```python
from build123d import *

# Parameters (mm, degrees)
SKETCH_W     = 10
SKETCH_H     = 10
PAD_DEPTH    = 2
SKETCH001_W  = 10
SKETCH001_H  = 10
PAD001_DEPTH = 2
SKETCH002_R  = 2.45
PAD002_DEPTH = 3.8
FILLET_R     = 2


with BuildPart() as part:
    # Sketch → Pad (new body)
    with BuildSketch(Plane.XY):
        Rectangle(SKETCH_W, SKETCH_H)
    extrude(amount=PAD_DEPTH)

    # Sketch001 (on Face3 of Pad) → Pad001 (join)
    with BuildSketch(Plane.XZ.offset(5)):
        with Locations((0, 5)):
            Rectangle(SKETCH001_W, SKETCH001_H)
    extrude(amount=PAD001_DEPTH)

    # Sketch002 → Pad002 (join)
    with BuildSketch(Plane.XZ.offset(7)):
        with Locations((0, 5)):
            Circle(SKETCH002_R)
    extrude(amount=PAD002_DEPTH)

    # Fillet
    fillet_edges = [part.edges().sort_by_distance(p)[0] for p in [
        (0, -5, 2),
    ]]
    fillet(fillet_edges, radius=FILLET_R)


solid = part.part
```
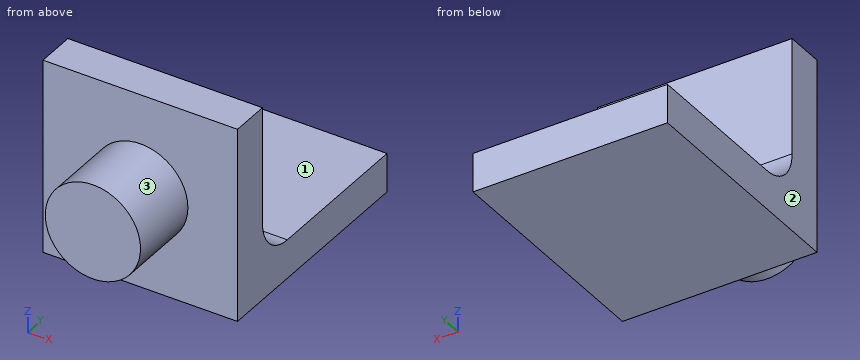
Could you check a few things on this model? Use its own coordinates, in mm. Face numbers are marked on the shaded views. A direction names the side the tool comes from. Coordinates: 2 decimals unless noted, no trailing zeros. Order: outer loops, then holes, each group sorted by start corner. A loop starts at its lowest first (then second) coordinate and runs counter-clockwise, first axis right, second up. Notation, with made-up numbers: M 40,59.5 L 54,59.5 A33 cw 54,97.5 Z; hole C 26,79.5 d2. An arc over 180 degrees is marked long. Use a Markdown table: item, result. Add a question column.
Q1. If I drill on L1, parallel to Y at x = -1, z = 5; L2, parallel to Y at x = 2.5, z = 5; L3, parallel to Z at x = 1, y = -2.5, over which ranges is the centre line in solid material (lowest first)?
Q2. I want a section at D-D on x = 0. List the corners of the cut face in (y, z) for me.
Q3. I'm going to push flat-ended pins straight in: pin 1 (2 mm diameter, centred on x = 1.5, y = -2.5, fed in from +Z); pin 2 (6 mm diameter, centred on x = -1.5, z = 8.5, fed in from +Y). Where does each tip first touch, or does it pass through?
Q4. I want a section at A-A on x = -4.25. List the corners of the cut face in (y, z) for me.
Q5. I want a section at C-C on y = 1.25. List the corners of the cut face in (x, z) for me.
Q6. I want a section at B-B on z = 5. List the corners of the cut face in (x, y) for me.
Q7. Which directions (+Z, -Z, +X, -X, +Y, -Y) give clear straight access to the entire face, cutting with the end or side of a thin tool? Please do the marked faces 1, 2 and 3.
Checked values:
| question | item | result |
|---|---|---|
| 1 | L1 | -10.8 to -5 |
| 1 | L2 | -7 to -5 |
| 1 | L3 | 0 to 2 |
| 2 | outline | M -10.8,2.55 L -7,2.55 L -7,0 L 5,0 L 5,2 L -3,2 A2 cw -5,4 L -5,10 L -7,10 L -7,7.45 L -10.8,7.45 Z |
| 3 | pin 1 | z = 2.06 |
| 3 | pin 2 | y = -5 |
| 4 | outline | M -7,0 L 5,0 L 5,2 L -3,2 A2 cw -5,4 L -5,10 L -7,10 Z |
| 5 | outline | M -5,0 L 5,0 L 5,2 L -5,2 Z |
| 6 | outline | M -5,-7 L -2.45,-7 L -2.45,-10.8 L 2.45,-10.8 L 2.45,-7 L 5,-7 L 5,-5 L -5,-5 Z |
| 7 | face 1 | +Z, +X, -X, +Y |
| 7 | face 2 | +Z, -Z, -X, +Y, -Y |
| 7 | face 3 | -Y |
